```python
from build123d import *

# Parameters (mm, degrees)
F1_DEPTH = 8
F2_R     = 3.99999
F3_R     = 1.75
F4_DEPTH = 4.5
F5_R     = 1.75
F6_DEPTH = 4.84


# Not quite as in the source:
# - a fillet or chamfer is up to 0.001 mm smaller than in the source, because OpenCascade refuses the exact size
# - a feature names something its author has since deleted; it is built from what else it names


with BuildPart() as f1:
    # F0 (on Top) → F1 (new body)
    with BuildSketch(Plane.XY):
        Polygon((4.5, 0), (0, 0), (0, -21), (7.7216494845, -26.6237113402), (10.7371134021, -23.2835051546), (4.5, -19), align=None)
    extrude(amount=F1_DEPTH)

    # F2 (radius 4 in the source; OpenCascade refuses exactly that, so slightly less here)
    f2_edges = [f1.edges().sort_by_distance(p)[0] for p in [
        (2.25, 0, 8),
        (2.25, 0, 0),
    ]]
    fillet(f2_edges, radius=F2_R)

    # F3 (on face) → F4 (cut)
    with BuildSketch(Plane.YZ.offset(4.5)):
        with Locations((-4, 4)):
            Circle(F3_R)
    extrude(amount=-F4_DEPTH, mode=Mode.SUBTRACT)

    # F5 (on face) → F6 (cut)
    with BuildSketch(Plane(origin=(-7.4244465835, -10.8105660241, 0), x_dir=(-0.8243201098, 0.5661239763, 0), z_dir=(0.5661239763, 0.8243201098, 0))):
        with Locations((-18.248982531, 4)):
            Circle(F5_R)
    extrude(amount=-F6_DEPTH, mode=Mode.SUBTRACT)


solid = f1.part
```
Model file for the job. Use its own axes, mm. Coordinates: 2 decimals unless noted, no trailing zeros. Order: outer loops, then holes, each group sorted by start corner. A loop starts at its lowest first (then second) coordinate and runs counter-clockwise, first axis right, second up. Notation, with made-up numbers: (23, 50) -> (29, 50) arc R32 cw to (29, 80) -> close; hole circle Ø11 at (-1.75, 26). An arc over 180 degrees is marked (long way). Answer as a JSON object with one key per item and string values. Group by question number.
1) Cut at C-C, the plane z = 7.75. Write the cut outline in (x, y).
2) Cut at D-D, the plane z = 0.75. Write the cut outline in (x, y).
3) Cut at B-B, the plane y = -17.5. Write the cut outline in (x, z).
4) Cut at A-A, the plane z = 4.5. Write the cut outline in (x, y), then the cut area to 3 significant figures.
5) Pull direction Y, two halves, no side cores. Call faces 1 (the face through (2.28, -5.39, 2.94)), 2 (the face through (4.5, -10, 4)), 3 (the face through (2.218, -1.141, 1.203)), 4 (the face through (5.719, -22.481, 2.447)): +Y half, -Y half, draft (parallel to the pull), parting line (faces both ways), or undercut.
6) Flat gauge pins, fed straight in: pin 1 (4 mm diameter, centred on x = 1.5, z = 1, fed in from +Y); pin 2 (1.5 mm diameter, centred on y = -22, z = 2.5, fed in from +X). Where does each tip first touch, or does it go through?
7) Drill centre lines: L1, parallel to Z at x = 2, y = -4; L2, parallel to X at y = -3, z = 2.5; L3, parallel to Z at x = 1.25, y = -1.75. Where is each one in solid material? Low to high.
Check values:
{
 "1": {"outline": "(0, -21) -> (7.72, -26.62) -> (10.74, -23.28) -> (4.5, -19) -> (4.5, -2.61) -> (0, -2.61) -> close"},
 "2": {"outline": "(0, -21) -> (7.72, -26.62) -> (10.74, -23.28) -> (4.5, -19) -> (4.5, -1.67) -> (0, -1.67) -> close"},
 "3": {"outline": "(0, 0) -> (4.5, 0) -> (4.5, 8) -> (0, 8) -> close"},
 "4": {"outline": "(0, -21) -> (3.79, -23.76) -> (6.24, -20.19) -> (4.5, -19) -> (4.5, -5.68) -> (0, -5.68) -> close; (0, -2.32) -> (4.5, -2.32) -> (4.5, -0.03) -> (0, -0.03) -> close; (6.5, -25.73) -> (7.72, -26.62) -> (10.74, -23.28) -> (9, -22.09) -> close", "area": "97.4 mm²"},
 "5": {"face 1": "undercut", "face 2": "draft", "face 3": "+Y half", "face 4": "undercut"},
 "6": {"pin 1": "stops at y = -0.13", "pin 2": "stops at x = 9.96"},
 "7": {"L1": "z = 0 to 2.25, 5.75 to 8", "L2": "x = 0 to 4.5", "L3": "z = 0.69 to 7.31"}
}
